from build123d import *

# Parameters (mm, degrees)
SKETCH1_R           = 25.4
SKETCH1_R_2         = 9.525
BOSS_EXTRUDE1_DEPTH = 12.7
FILLET1_R           = 12.7


with BuildPart() as part:
    # Sketch1 → Boss-Extrude1 (new body)
    with BuildSketch(Plane(origin=(0, 0, 0), x_dir=(1, 0, 0), z_dir=(0, 1, 0))):
        with BuildLine():
            Line((-24.35791626, 29.296790191), (-19.05, 59.399479175))
            ThreePointArc((-19.05, 59.399479175), (0, 101.6), (19.05, 59.399479175))
            Line((19.05, 59.399479175), (24.35791626, 29.296790191))
            ThreePointArc((24.35791626, 29.296790191), (0, -38.1), (-24.35791626, 29.296790191))
        make_face()
        with Locations(Location((0, 0, 0), (0, 0, 270))):
            Circle(SKETCH1_R, mode=Mode.SUBTRACT)
        with Locations(Location((0, 76.2, 0), (0, 0, 270))):
            Circle(SKETCH1_R_2, mode=Mode.SUBTRACT)
    extrude(amount=BOSS_EXTRUDE1_DEPTH)

    # Fillet1
    fillet1_edges = [part.edges().sort_by_distance(p)[0] for p in [
        (19.05, 6.35, -59.399479175),
        (24.35791626, 6.35, -29.296790191),
        (-24.35791626, 6.35, -29.296790191),
        (-19.05, 6.35, -59.399479175),
    ]]
    fillet(fillet1_edges, radius=FILLET1_R)


solid = part.part
Could you check a few things on this model? Use its own coordinates, in mm. A direction names the side the tool comes from. Give positions to 0.01 mm unless a question says otherwise; leave off trailing zeros. Order: outer loops, then holes, each group sorted by start corner. A loop starts at its lowest first (then second) coordinate and runs counter-clockwise, first axis right, second up. Notation, with made-up numbers: (3.25, -36) - (16.25, -36) arc R23 ccw to (16.25, -5) - close; hole circle Ø5 at (4, 36). An arc over 180 degrees is marked (long way). One line per question, with ' | ' between items. Start each with the question number.
Item 1: I need wall thicknesses on probe 1 along X at (y, z) = (9.25, -76.2) (3 decimals); probe 2 along X at (y, z) = (10, 0); probe 3 along Z at (x, y) = (-4, 5.5). Which ranges of each line are inside material? Lowest first, please. Write a range as [from, to].
Item 2: For faces 1 (the cylindrical face through (-24.82, 6.44, -29.93)), 2 (the cylindrical face through (-15.456, 6.261, -20.157)), 3 (the cylindrical face through (24.865, 6.439, -29.839)), which set-ups out of +Z, -Z, +X, -X, +Y, -Y let a thin tool reach every point of the face, with its end or its side?
Item 3: Thinking about a two-plate mould opening in Z: for faces 4 (the cylindrical face through (1.25, 6.26, 38.08)), 5 (the flat face through (1, 0, -33)), 6 (the cylindrical face through (20.027, 6.439, -58.733)), 7 (the cylindrical face through (-0.75, 6.26, -101.59)), which applies, pulls with the +Z half, pulls with the -Z half, needs draft (parallel to the pull), parting line crosses it, or undercut?
Item 4: I want a section at D-D on z = -36.5. Write out the boundary of the cut face in (x, y).
Item 5: I want a section at A-A on z = -76.2. Write out the boundary of the cut face in (x, y) (3 decimals), then the cut area to 3 significant figures.
Item 6: I want a section at B-B on y = 5.5. Write out the boundary of the cut face in (x, z) (3 decimals), then the cut area to 3 significant figures.
Item 7: I'm going to push flat-ended pins straight in: pin 1 Ø1.5 at (y, z) = (10, -28.5) entering from -X; pin 2 Ø1 at (x, y) = (-7, 3) entering from +Z. Where does each tip first touch, or does it pass through?
Item 8: I want a section at C-C on x = -16.5. Write out the boundary of the cut face in (y, z), then the cut area to 3 significant figures.
Verdict:
1) probe 1: [-25.4, -9.525], [9.525, 25.4] | probe 2: [-38.1, -25.4], [25.4, 38.1] | probe 3: [-101.28, -84.84], [-67.56, -25.08], [25.08, 37.89]
2) face 1: -X, +Y, -Y | face 2: +Y, -Y | face 3: +X, +Y, -Y
3) face 4: parting line crosses it | face 5: needs draft | face 6: undercut | face 7: undercut
4) outline: (-23.09, 0) - (23.09, 0) - (23.09, 12.7) - (-23.09, 12.7) - close
5) outline: (-25.4, 0) - (-9.525, 0) - (-9.525, 12.7) - (-25.4, 12.7) - close; (9.525, 0) - (25.4, 0) - (25.4, 12.7) - (9.525, 12.7) - close | area: 403 mm^2
6) outline: (-27.091, -26.79) arc R12.7 cw to (-23.614, -33.514) - (-19.985, -54.098) arc R12.7 cw to (-21.661, -62.935) arc R25.4 ccw (long way) to (21.661, -62.935) arc R12.7 cw to (19.985, -54.098) - (23.614, -33.514) arc R12.7 cw to (27.091, -26.79) arc R38.1 ccw (long way) to start; hole circle Ø50.8 at (0, 0); hole circle Ø19.05 at (0, -76.2) | area: 5,070 mm^2
7) pin 1: x = -26.23 | pin 2: z = 37.54
8) outline: (0, -95.51) - (12.7, -95.51) - (12.7, -19.31) - (0, -19.31) - close; (0, 19.31) - (12.7, 19.31) - (12.7, 34.34) - (0, 34.34) - close | area: 1,160 mm^2
